from build123d import *

# Parameters (mm, degrees)
F0_W     = 50
F0_H     = 25
F1_DEPTH = 25
F2_R     = 6.25
F3_DEPTH = 10
F5_D     = 4.1
F6_T     = -1


with BuildPart() as f1:
    # F0 (on Top) → F1 (new body)
    with BuildSketch(Plane.XY):
        Rectangle(F0_W, F0_H)
    extrude(amount=F1_DEPTH)

    # F2 (on face) → F3 (cut)
    with BuildSketch(Plane.XY.offset(25)):
        with Locations((12, 1.5)):
            Circle(F2_R)
    extrude(amount=-F3_DEPTH, mode=Mode.SUBTRACT)

    # F5 (through all)
    with Locations(Plane.XY.offset(25)):
        with Locations((-14.193482697, -5.1824725233)):
            Hole(F5_D / 2)

    # F6
    f6_openings = [f1.faces().sort_by_distance(p)[0] for p in [
        (0.151512, 0.055322, 0),
    ]]
    offset(amount=F6_T, openings=f6_openings, kind=Kind.INTERSECTION)


solid = f1.part
Can you work these out from the model? Positions are in its coordinate system, mm. A direction names the side the tool comes from. Give positions to 0.01 mm unless a question says otherwise; leave off trailing zeros. Loops run counter-clockwise (first coordinate to the right, second up) from the corner with the lowest first, then second, coordinate; pieces in that order, holes last. Notation, with made-up numbers: M 29.25,20 L 67.25,20 A17 cw 67.25,40 Z; hole C 43.25,45 d4. An arc over 180 degrees is marked long. One line per item, written item: value. Start each with the question number.
1) Thinking about a two-plate mould opening in Y: for faces 1 (the face through (0, -12.5, 12)), 2 (the face through (0, 0, 25)), 3 (the face through (0, 0, 24)), which applies, +Y half, -Y half, draft (parallel to the pull), parting line (faces both ways), or undercut?
2) If we section it at B-B, the plane y = -9: Write out the boundary of the cut face in (x, z), and give its area (3 significant figures).
3) If we section it at C-C, the plane z = 11.5: Write out the boundary of the cut face in (x, y).
4) If I drill on line 1 (Y direction, x = 12, z = 23.25); line 2 (X direction, y = 6, z = 10); line 3 (Y direction, x = -17.5, z = 13.5), over which ranges is the centre line in solid material (lowest first)? Write a range as [from, to].
5) If we section it at D-D, the plane x = 12: Write out the boundary of the cut face in (y, z).
6) I'm going to push flat-ended pins straight in: pin 1 (3.5 mm diameter, centred on x = -14.19, y = -5.18, fed in from +Z); pin 2 (3 mm diameter, centred on x = 11.5, y = 6.5, fed in from -Z); pin 3 (2 mm diameter, centred on x = -10, y = 8, fed in from -Z). Where does each tip first touch, or does it pass through?
7) If we section it at A-A, the plane z = 16.25: Write out the boundary of the cut face in (x, y), and give its area (3 significant figures).
8) On a 3-axis mill with a long thin cutter (end or side, diameter ignored), from which of +Z, -Z, +X, -X, +Y, -Y can I reach the whole of each face in a straight line? I mean faces 4 (the face through (0, 12.5, 12)), 5 (the face through (7.39, 5.72, 20.07)), 6 (the face through (-15.83, -2.61, 11.83)). Say none if no direction works.
Completed:
1. face 1: -Y half
1. face 2: draft
1. face 3: undercut
2. outline: M -25,0 L -24,0 L -24,24 L 24,24 L 24,0 L 25,0 L 25,25 L -25,25 Z
2. area: 98.0 mm^2
3. outline: M -25,-12.5 L 25,-12.5 L 25,12.5 L -25,12.5 Z; C -14.19,-5.18 d6.1; hole M -24,-11.5 L 24,-11.5 L 24,11.5 L -24,11.5 Z; hole C -14.19,-5.18 d4.1
4. line 1: y = [-12.5, -11.5], [-5.75, -4.75], [7.75, 8.75], [11.5, 12.5]
4. line 2: x = [-25, -24], [24, 25]
4. line 3: y = [-12.5, -11.5], [11.5, 12.5]
5. outline: M -12.5,0 L -11.5,0 L -11.5,24 L -5.75,24 L -5.75,14 L 8.75,14 L 8.75,24 L 11.5,24 L 11.5,0 L 12.5,0 L 12.5,25 L 7.75,25 L 7.75,15 L -4.75,15 L -4.75,25 L -12.5,25 Z
6. pin 1: passes through
6. pin 2: stops at z = 14
6. pin 3: stops at z = 24
7. outline: M -25,-12.5 L 25,-12.5 L 25,12.5 L -25,12.5 Z; C -14.19,-5.18 d6.1; C 12,1.5 d14.5; hole M -24,-11.5 L 24,-11.5 L 24,11.5 L -24,11.5 Z; hole C -14.19,-5.18 d4.1; hole C 12,1.5 d12.5
7. area: 204 mm^2
8. face 4: +Z, -Z, +X, -X, +Y
8. face 5: +Z
8. face 6: -Z
